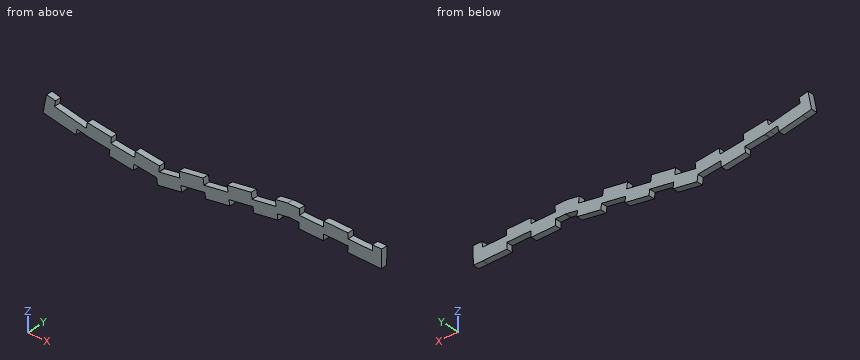
```python
from build123d import *

# Parameters (mm, degrees)
F1_DEPTH = 3.27


with BuildPart() as f1:
    # F0 (on Front) → F1 (new body)
    with BuildSketch(Plane.XZ):
        Polygon((88.0849202076, -6.1928071498), (88.0849202076, -2.9228071498), (84.155737444, -2.8377134103), (84.0849513189, -6.1062455567), align=None)
        Polygon((84.155737444, -2.8377134103), (88.0849202076, -2.9228071498), (88.0849202076, -6.1928071498), (84.0849513189, -6.1062455567), (84.0164814126, -9.2678268597), (88.8164814126, -9.3717797613), (89.0171933904, -0.1039529016), (84.2171933904, 0), align=None)
        Polygon((84.0849513189, -6.1062455567), (84.155737444, -2.8377134103), (71.4586099838, -2.5627335684), (71.387872598, -5.8314735793), align=None)
        Polygon((71.387872598, -5.8314735793), (71.4586099838, -2.5627335684), (58.7615872094, -2.2877559936), (58.6908453502, -5.5567027157), align=None)
        Polygon((58.7615872094, -2.2877559936), (71.4586099838, -2.5627335684), (71.5200152581, 0.27477413), (58.8229924837, 0.5497517048), align=None)
        Polygon((84.0164814126, -9.2678268597), (84.0849513189, -6.1062455567), (71.387872598, -5.8314735793), (71.3194541632, -8.9930559962), align=None)
        Polygon((58.6908453502, -5.5567027157), (58.7615872094, -2.2877559936), (46.0645644334, -2.0127784187), (45.9938181008, -5.2819318522), align=None)
        with BuildLine():
            Line((45.9938181008, -5.2819318522), (46.0645644334, -2.0127784187))
            Line((46.0645644334, -2.0127784187), (41.0805670131, -1.9048407118))
            ThreePointArc((41.0805670131, -1.9048407118), (40.5264072315, -1.9163330219), (39.9752108165, -1.9747080916))
            Line((39.9752108165, -1.9747080916), (33.9712176037, -2.8692401974))
            Line((33.9712176037, -2.8692401974), (34.4530943895, -6.1035399305))
            Line((34.4530943895, -6.1035399305), (40.4570876022, -5.2090078247))
            ThreePointArc((40.4570876022, -5.2090078247), (40.7326592445, -5.1798219691), (41.0097124764, -5.1740729826))
            Line((41.0097124764, -5.1740729826), (45.9938181008, -5.2819318522))
        make_face()
        with BuildLine():
            Line((41.0805670131, -1.9048407118), (46.0645644334, -2.0127784187))
            Line((46.0645644334, -2.0127784187), (46.1317693836, 1.0927294697))
            Line((46.1317693836, 1.0927294697), (39.9752108165, 1.2259608853))
            Line((39.9752108165, 1.2259608853), (33.5047069945, 0.2619235848))
            Line((33.5047069945, 0.2619235848), (33.9712176037, -2.8692401974))
            Line((33.9712176037, -2.8692401974), (39.9752108165, -1.9747080916))
            ThreePointArc((39.9752108165, -1.9747080916), (40.5264072315, -1.9163330219), (41.0805670131, -1.9048407118))
        make_face()
        Polygon((58.6224313888, -8.7180784214), (58.6908453502, -5.5567027157), (45.9938181008, -5.2819318522), (45.9254041394, -8.4433075578), align=None)
        Polygon((34.4530943895, -6.1035399305), (33.9712176037, -2.8692401974), (21.4098700166, -4.7407494263), (21.8917468023, -7.9750491594), align=None)
        Polygon((21.8917468023, -7.9750491594), (21.4098700166, -4.7407494263), (8.8485224294, -6.6122586553), (9.3303992151, -9.8465583884), align=None)
        Polygon((8.8485224294, -6.6122586553), (21.4098700166, -4.7407494263), (20.9433594073, -1.6095856442), (8.3820118202, -3.4810948731), align=None)
        Polygon((34.8707613687, -8.9068710714), (34.4530943895, -6.1035399305), (21.8917468023, -7.9750491594), (22.3094137815, -10.7783803003), align=None)
        Polygon((9.3303992151, -9.8465583884), (8.8485224294, -6.6122586553), (-3.7128251578, -8.4837678842), (-3.2309483721, -11.7180676173), align=None)
        Polygon((-3.2309483721, -11.7180676173), (-3.7128251578, -8.4837678842), (-16.274172745, -10.3552771132), (-15.7922959593, -13.5895768463), align=None)
        Polygon((-16.274172745, -10.3552771132), (-3.7128251578, -8.4837678842), (-4.179335767, -5.3526041021), (-16.7406833542, -7.224113331), align=None)
        Polygon((9.7480661944, -12.6498895293), (9.3303992151, -9.8465583884), (-3.2309483721, -11.7180676173), (-2.8132813928, -14.5213987582), align=None)
        with BuildLine():
            Line((-15.7922959593, -13.5895768463), (-16.274172745, -10.3552771132))
            Line((-16.274172745, -10.3552771132), (-26.8291325696, -11.9278555795))
            ThreePointArc((-26.8291325696, -11.9278555795), (-27.0463868948, -11.9528310654), (-27.2648247248, -11.9632296803))
            Line((-27.2648247248, -11.9632296803), (-27.3333623041, -12.5313407106))
            Line((-27.3333623041, -12.5313407106), (-27.6582478154, -15.224331103))
            ThreePointArc((-27.6582478154, -15.224331103), (-27.0011881523, -15.2262131022), (-26.3472557839, -15.1621553125))
            Line((-26.3472557839, -15.1621553125), (-15.7922959593, -13.5895768463))
        make_face()
        with BuildLine():
            Line((-15.350207165, -16.5568243078), (-15.7922959593, -13.5895768463))
            Line((-15.7922959593, -13.5895768463), (-26.3472557839, -15.1621553125))
            ThreePointArc((-26.3472557839, -15.1621553125), (-27.0011881523, -15.2262131022), (-27.6582478154, -15.224331103))
            ThreePointArc((-27.6582478154, -15.224331103), (-27.8766021467, -15.2090531255), (-28.0943229104, -15.186476597))
            Line((-28.0943229104, -15.186476597), (-28.4000527535, -15.1495929911))
            Line((-28.4000527535, -15.1495929911), (-27.9115547522, -18.4283335368))
            Line((-27.9115547522, -18.4283335368), (-15.350207165, -16.5568243078))
        make_face()
        with BuildLine():
            Line((-27.3333623041, -12.5313407106), (-27.2648247248, -11.9632296803))
            ThreePointArc((-27.2648247248, -11.9632296803), (-27.4841349376, -11.9589696843), (-27.7026661329, -11.9400162217))
            Line((-27.7026661329, -11.9400162217), (-39.8769224488, -10.4712996977))
            Line((-39.8769224488, -10.4712996977), (-40.2685792263, -13.717760073))
            Line((-40.2685792263, -13.717760073), (-28.4000527535, -15.1495929911))
            Line((-28.4000527535, -15.1495929911), (-28.0943229104, -15.186476597))
            ThreePointArc((-28.0943229104, -15.186476597), (-27.8766021467, -15.2090531255), (-27.6582478154, -15.224331103))
            Line((-27.6582478154, -15.224331103), (-27.3333623041, -12.5313407106))
        make_face()
        with BuildLine():
            ThreePointArc((-27.7026661329, -11.9400162217), (-27.4841349376, -11.9589696843), (-27.2648247248, -11.9632296803))
            Line((-27.2648247248, -11.9632296803), (-26.9090273113, -9.0140091622))
            Line((-26.9090273113, -9.0140091622), (-39.5176043042, -7.4928956836))
            Line((-39.5176043042, -7.4928956836), (-39.8769224488, -10.4712996977))
            Line((-39.8769224488, -10.4712996977), (-27.7026661329, -11.9400162217))
        make_face()
        Polygon((-40.2685792263, -13.717760073), (-39.8769224488, -10.4712996977), (-52.3508780033, -8.9664271069), (-52.3940183108, -8.9612226097), (-52.8326980236, -12.2020100831), align=None)
        Polygon((-52.3940183108, -8.9612226097), (-52.3508780033, -8.9664271069), (-51.9915598587, -5.9880230928), align=None)
        Polygon((-40.6498897454, -16.8784598537), (-40.2685792263, -13.717760073), (-52.8326980236, -12.2020100831), (-53.2351142651, -15.1748977649), align=None)
        with BuildLine():
            Line((-52.8326980236, -12.2020100831), (-52.3940183108, -8.9612226097))
            Line((-52.3940183108, -8.9612226097), (-62.6937612549, -7.7186495717))
            ThreePointArc((-62.6937612549, -7.7186495717), (-62.824652475, -7.7001674476), (-62.9546897587, -7.6764102329))
            Line((-62.9546897587, -7.6764102329), (-65.1754864714, -7.224113331))
            Line((-65.1754864714, -7.224113331), (-65.8285059402, -10.4298488094))
            Line((-65.8285059402, -10.4298488094), (-63.6028382914, -10.8815332771))
            ThreePointArc((-63.6028382914, -10.8815332771), (-63.3449657453, -10.9285070615), (-63.0854180325, -10.9651099471))
            Line((-63.0854180325, -10.9651099471), (-52.8326980236, -12.2020100831))
        make_face()
        with BuildLine():
            Line((-62.6937612549, -7.7186495717), (-52.3940183108, -8.9612226097))
            Line((-52.3940183108, -8.9612226097), (-51.9915598587, -5.9880230928))
            Line((-51.9915598587, -5.9880230928), (-64.5767843783, -4.284461004))
            Line((-64.5767843783, -4.284461004), (-65.1754864714, -7.224113331))
            Line((-65.1754864714, -7.224113331), (-62.9546897587, -7.6764102329))
            ThreePointArc((-62.9546897587, -7.6764102329), (-62.824652475, -7.7001674476), (-62.6937612549, -7.7186495717))
        make_face()
        Polygon((-65.8285059402, -10.4298488094), (-65.1754864714, -7.224113331), (-81.7354778523, -3.8514350694), (-82.3907114007, -7.0686592077), (-69.9444316109, -9.5945490301), align=None)
        Polygon((-86.2950797924, -2.9228071498), (-81.7354778523, -3.8514350694), (-81.1461729514, -0.9579233488), (-85.8496166746, 0), (-87.7128069895, -9.1483424039), (-83.0093632663, -10.1062657528), (-82.3907114007, -7.0686592077), (-86.2950797924, -6.2762935732), align=None)
        Polygon((-82.3907114007, -7.0686592077), (-81.7354778523, -3.8514350694), (-86.2950797924, -2.9228071498), (-86.2950797924, -6.2762935732), align=None)
        Polygon((-69.9444316109, -9.5945490301), (-82.3907114007, -7.0686592077), (-83.0093632663, -10.1062657528), (-70.5410984981, -12.5346151222), align=None)
    extrude(amount=F1_DEPTH)


solid = f1.part
```
The listing builds one solid part. Answer for the finished solid, in the listing's coordinates (mm). Give positions to 0.01 mm unless a question says otherwise; leave off trailing zeros. Loops run counter-clockwise (first coordinate to the right, second up) from the corner with the lowest first, then second, coordinate; pieces in that order, holes last. Notation, with made-up numbers: (12.5, 17.25) - (24.5, 17.25) arc R8 ccw to (24.5, 22.25) - close; hole circle Ø4 at (41, 82.5). An arc over 180 degrees is marked (long way). Return JSON: item names as keys, results as strings. Group by question number.
1. Find section B-B (x = -61). Write down the section's boundary in (y, z).
2. Find section A-A (x = 56). Write down the section's boundary in (y, z), then the cut area to 3 significant figures.
3. Straight lines are drawn through the part: line 1 (X direction, y = -0.65, z = -1); line 2 (Z direction, x = 74.5, y = -2.65); line 3 (Z direction, x = 33, y = -1.75). For each, find the intervals that lie inside material, in ascending order. Write a range as [from, to].
Verdict:
{
 "1": {"outline": "(-3.27, -11.22) - (0, -11.22) - (0, -4.77) - (-3.27, -4.77) - close"},
 "2": {"outline": "(-3.27, -8.66) - (0, -8.66) - (0, -2.23) - (-3.27, -2.23) - close", "area": "21.0 mm^2"},
 "3": {"line 1": "x = [-86.05, -81.15], [33.69, 46.09], [58.79, 71.49], [84.2, 89]", "line 2": "z = [-9.06, -2.63]", "line 3": "z = [-9.19, -3.01]"}
}
